Geometry check sheet. Reference: the model listing, model coordinates, mm. A direction names the side the tool comes from. Round coordinates to 2 decimals unless told otherwise and drop trailing zeros. Order: outer loops, then holes, each group sorted by start corner. A loop starts at its lowest first (then second) coordinate and runs counter-clockwise, first axis right, second up.
```python
from build123d import *

# Parameters (mm, degrees)
SKETCH1_W             = 42
SKETCH1_H             = 42
BOSS_EXTRUDE1_DEPTH   = 6.35
M3_CLEARANCE_HOLE1_D  = 3.2
SKETCH6_R             = 11.5
CUT_EXTRUDE1_DEPTH    = 7.35
BOSS_EXTRUDE2_DEPTH   = 6.35
F_6_CLEARANCE_HOLE1_D = 3.6576
CIRPATTERN2_COUNT     = 4
FILLET2_R             = 3


with BuildPart() as part:
    # Sketch1 → Boss-Extrude1 (new body)
    with BuildSketch(Plane(origin=(0, 0, 0), x_dir=(1, 0, 0), z_dir=(0, 1, 0))):
        Rectangle(SKETCH1_W, SKETCH1_H)
    extrude(amount=BOSS_EXTRUDE1_DEPTH)

    # M3 Clearance Hole1 (through all)
    with Locations(Plane(origin=(0, 6.35, 0), x_dir=(1, 0, 0), z_dir=(0, 1, 0))):
        with Locations((-15.5, 15.5), (-15.5, -15.5), (15.5, -15.5), (15.5, 15.5)):
            Hole(M3_CLEARANCE_HOLE1_D / 2)

    # Sketch6 → Cut-Extrude1 (cut, through all)
    with BuildSketch(Plane(origin=(0, 6.35, 0), x_dir=(1, 0, 0), z_dir=(0, 1, 0))):
        Circle(SKETCH6_R)
    extrude(amount=-CUT_EXTRUDE1_DEPTH, mode=Mode.SUBTRACT)

    # Sketch7 → Boss-Extrude2 (add)
    with BuildSketch(Plane(origin=(0, 6.35, 0), x_dir=(1, 0, 0), z_dir=(0, 1, 0))):
        with BuildLine():
            Line((-25.535533906, 18.464466094), (-21, 13.928932188))
            Line((-21, 13.928932188), (-21, 21))
            Line((-21, 21), (-13.928932188, 21))
            Line((-13.928932188, 21), (-18.464466094, 25.535533906))
            ThreePointArc((-18.464466094, 25.535533906), (-25.535533906, 25.535533906), (-25.535533906, 18.464466094))
        make_face()
    boss_extrude2 = extrude(amount=-BOSS_EXTRUDE2_DEPTH)

    # 6 Clearance Hole1 (through all)
    with Locations(Plane(origin=(0, 6.35, 0), x_dir=(1, 0, 0), z_dir=(0, 1, 0))):
        with Locations((-22, 22)):
            f_6_clearance_hole1 = Hole(F_6_CLEARANCE_HOLE1_D / 2)

    # CirPattern2: Boss-Extrude2, 6 Clearance Hole1 ×4 about axis
    cirpattern2_axis = Axis((0, 0, 0), (0, 1, 0))
    for i in range(1, CIRPATTERN2_COUNT):
        add(boss_extrude2.rotate(cirpattern2_axis, i * 360 / CIRPATTERN2_COUNT))
        add(f_6_clearance_hole1.rotate(cirpattern2_axis, i * 360 / CIRPATTERN2_COUNT), mode=Mode.SUBTRACT)

    # Fillet2
    fillet2_edges = [part.edges().sort_by_distance(p)[0] for p in [
        (-13.928932188, 3.175, -21),
        (-21, 3.175, -13.928932188),
        (-21, 3.175, 13.928932188),
        (-13.928932188, 3.175, 21),
        (13.928932188, 3.175, 21),
        (21, 3.175, 13.928932188),
        (21, 3.175, -13.928932188),
        (13.928932188, 3.175, -21),
    ]]
    fillet(fillet2_edges, radius=FILLET2_R)


solid = part.part
```
(1) Sectioned sample at C-C, the plane y = 5.5. Give the number of separate pieces and of enclosed holes in the cut face, and give its area (3 significant figures).
Returned:
separate pieces: 1
enclosed holes: 9
area: 1,590 mm2
(2) Sectioned sample at A-A, the plane x = 0. Record the cut outline in (y, z), and give its area (3 significant figures).
Returned:
outline: (0, -21) - (6.35, -21) - (6.35, -11.5) - (0, -11.5) - close; (0, 11.5) - (6.35, 11.5) - (6.35, 21) - (0, 21) - close
area: 121 mm2
(3) Sectioned sample at B-B, the plane z = 0. Record the cut outline in (x, y), and give its area (3 significant figures).
Returned:
outline: (-21, 0) - (-11.5, 0) - (-11.5, 6.35) - (-21, 6.35) - close; (11.5, 0) - (21, 0) - (21, 6.35) - (11.5, 6.35) - close
area: 121 mm2
(4) Draft check along X on faces 1 (the cylindrical face through (-21.222, 3.131, 13.819)), 2 (the cylindrical face through (22.549, 3.131, -23.744)), 3 (the flat face through (23.68, 3.22, -16.61)), 4 (the cylindrical face through (23.744, 3.131, 22.549)). Enter one of: released by +X, released by -X, zero draft, split by the parting line, or undercut.
Returned:
face 1: released by -X
face 2: undercut
face 3: released by +X
face 4: undercut
(5) Sectioned sample at D-D, the plane x = -15.5. Record the cut outline in (y, z), and give its area (3 significant figures).
Returned:
outline: (0, -22.57) - (6.35, -22.57) - (6.35, -17.1) - (0, -17.1) - close; (0, -13.9) - (6.35, -13.9) - (6.35, 13.9) - (0, 13.9) - close; (0, 17.1) - (6.35, 17.1) - (6.35, 22.57) - (0, 22.57) - close
area: 246 mm2
(6) Material ranges on line 1 (X direction, y = 6, z = 0); line 2 (X direction, y = 2.5, z = -15.5), recorded low to high.
Returned:
line 1: x = -21 to -11.5, 11.5 to 21
line 2: x = -22.57 to -17.1, -13.9 to 13.9, 17.1 to 22.57
(7) Depth check by flat-ended pin: P1, Ø1.5, axis at x = 13.5, y = 1.5, coming from the -Z side; P2, Ø2, axis at x = 5.5, y = 2.5, coming from the +Z side; P3, Ø1.5, axis at x = 13, y = 2, coming from the +Z side. Enter the tip coordinate at first touch or a pass-through.
Returned:
P1: stops at z = -21.44
P2: stops at z = 21
P3: stops at z = 21.19
(8) Set-up check for faces 5 (the flat face through (23.73, 3.22, 16.66)), 6 (the flat face through (16.66, 3.22, -23.73)), 7 (the flat face through (0, 0, 12)), 8 (the flat face through (0, 3, 21)), 9 (the flat face through (-21, 3, 0)): record each of +Z, -Z, +X, -X, +Y, -Y from which the full face is reachable in a straight line by a thin tool's end or side.
Returned:
face 5: +X, +Y, -Y
face 6: -Z, +Y, -Y
face 7: +Z, -Z, +X, -X, -Y
face 8: +Z, +Y, -Y
face 9: -X, +Y, -Y
